```python
from build123d import *

# Parameters (mm, degrees)
BOSS_EXTRUDE1_DEPTH     = 5
CUT_EXTRUDE1_REACH      = 9.033
CUT_EXTRUDE1_END_RADIUS = 2.5


with BuildPart() as part:
    # Sketch1 → Boss-Extrude1 (new body)
    with BuildSketch(Plane(origin=(0, 0, 0), x_dir=(1, 0, 0), z_dir=(0, 1, 0))):
        with BuildLine():
            Line((-1.767766953, -1.767766953), (1.767766953, -1.767766953))
            ThreePointArc((1.767766953, -1.767766953), (0, 2.5), (-1.767766953, -1.767766953))
        make_face()
    extrude(amount=BOSS_EXTRUDE1_DEPTH)

    # Cut-Extrude1: up to this cylinder (the profile starts inside it)
    cut_extrude1_end = Plane(origin=(0, 2.5, 0), z_dir=(0, -1, 0)) * Cylinder(CUT_EXTRUDE1_END_RADIUS, 27.887488, mode=Mode.PRIVATE)
    # Sketch2 → Cut-Extrude1 (cut, up to the surface)
    with BuildSketch(Plane.XY.offset(1.767766953), mode=Mode.PRIVATE) as cut_extrude1_sk1:
        Polygon((-1.767766953, 0), (0, 1.767766953), (1.767766953, 0), align=None)
    cut_extrude1_tool1 = extrude(cut_extrude1_sk1.sketch, amount=-CUT_EXTRUDE1_REACH, mode=Mode.PRIVATE) & cut_extrude1_end
    add(cut_extrude1_tool1.solids().sort_by_distance((0, 0.589256, 1.767767))[0], mode=Mode.SUBTRACT)
    # Sketch2 → Cut-Extrude1 (cut, up to the surface)
    with BuildSketch(Plane.XY.offset(1.767766953), mode=Mode.PRIVATE) as cut_extrude1_sk2:
        Polygon((-1.767766953, 5), (0, 3.232233047), (1.767766953, 5), align=None)
    cut_extrude1_tool2 = extrude(cut_extrude1_sk2.sketch, amount=-CUT_EXTRUDE1_REACH, mode=Mode.PRIVATE) & cut_extrude1_end
    add(cut_extrude1_tool2.solids().sort_by_distance((0, 4.410744, 1.767767))[0], mode=Mode.SUBTRACT)


solid = part.part
```
The listing builds one solid part. Answer for the finished solid, in the listing's coordinates (mm). A direction names the side the tool comes from. Give positions to 0.01 mm unless a question says otherwise; leave off trailing zeros. Loops run counter-clockwise (first coordinate to the right, second up) from the corner with the lowest first, then second, coordinate; pieces in that order, holes last. Notation, with made-up numbers: (6.25, 84) - (27.25, 84) arc R14 cw to (27.25, 110) - close; hole circle Ø8 at (32, 24). An arc over 180 degrees is marked (long way). Return JSON: item names as keys, results as strings. Group by question number.
1. Find section D-D (z = 0). Write down the section's boundary in (x, y).
2. Find section C-C (y = 1.85). Write down the section's boundary in (x, z), then the cut area to 3 significant figures.
3. Which of the six approach directions +Z, -Z, +X, -X, +Y, -Y give full straight-line access (tool end or side, diameter ignored) to faces 1 (the flat face through (0.87, 4.1, -0.34)), 2 (the flat face through (-0.9, 0.87, -0.34))?
4. Find section B-B (y = 4.65). Write down the section's boundary in (x, z), then the cut area to 3 significant figures.
5. Find section A-A (z = -0.7). Write down the section's boundary in (x, y), then the cut area to 4 significant figures.
6. Given pin 1 Ø2 at (x, y) = (-1, 4.5) entering from -Z, flat-ended and moving along its own axis, determine where the tip first touches the part or whether it passes through.
7. Straight lines are drawn through the part: line 1 (X direction, y = 4.4, z = -0.7); line 2 (X direction, y = 0.5, z = -1.95); line 3 (Z direction, x = -0.1, y = 2.5). For each, find the intervals that lie inside material, in ascending order. Write a range as [from, to].
8. Determine the mould class of faces 3 (the flat face through (0, 2, 1.768)), 4 (the cylindrical face through (0.1, 2.5, -2.5)), 5 (the flat face through (0.87, 0.9, -0.34)) for opening direction X: pulls with the +X half, pulls with the -X half, needs draft (parallel to the pull), parting line crosses it, or undercut.
Verdict:
{
 "1": {"outline": "(-2.5, 0) - (-1.77, 0) - (0, 1.77) - (1.77, 0) - (2.5, 0) - (2.5, 5) - (1.77, 5) - (0, 3.23) - (-1.77, 5) - (-2.5, 5) - close"},
 "2": {"outline": "(-1.77, 1.77) arc R2.5 ccw (long way) to (1.77, 1.77) - close", "area": "17.9 mm^2"},
 "3": {"face 1": "+Z, -Z, +Y", "face 2": "+Z, -Z, -Y"},
 "4": {"outline": "(-1.77, 1.77) arc R2.5 ccw to (-1.42, -2.06) - (-1.42, 1.77) - close; (1.42, -2.06) arc R2.5 ccw to (1.77, 1.77) - (1.42, 1.77) - close", "area": "6.15 mm^2"},
 "5": {"outline": "(-2.4, 0) - (-1.77, 0) - (0, 1.77) - (1.77, 0) - (2.4, 0) - (2.4, 5) - (1.77, 5) - (0, 3.23) - (-1.77, 5) - (-2.4, 5) - close", "area": "17.75 mm^2"},
 "6": {"pin 1": "stops at z = -2.46"},
 "7": {"line 1": "x = [-2.4, -1.17], [1.17, 2.4]", "line 2": "x = [-1.56, -1.27], [1.27, 1.56]", "line 3": "z = [-2.5, 1.77]"},
 "8": {"face 3": "needs draft", "face 4": "parting line crosses it", "face 5": "undercut"}
}
